Source: CAD feature listing. Evaluate the final solid. Frame: model axes, mm. Face numbers are marked on the shaded views. Coordinates: 2 decimals unless noted, no trailing zeros. Write each loop counter-clockwise with the first axis right and the second up, starting at its lowest first coordinate (ties: lowest second). Pieces come first, ordered by that corner, then holes. Notation, with made-up numbers: (-4, 56.25) -> (41, 56.25) arc R25 ccw to (41, 82.25) -> close; hole circle Ø6 at (79, 83). An arc over 180 degrees is marked (long way). One line per item, written item: value. Start each with the question number.
1. Line query: line 1 (Y direction, x = 0, z = 2.1); line 2 (X direction, y = -11, z = 0.5); line 3 (Z direction, x = 1.5, y = 17). Output: solid intervals per line, ascending.
2. Section query D-D, the plane x = 2.75. Output: boundary loops of the cut face in (y, z).
3. Section query B-B, the plane x = 0. Output: boundary loops of the cut face in (y, z).
4. Section query A-A, the plane y = 2.5. Output: boundary loops of the cut face in (x, z), and give its area (3 significant figures).
5. Mould query, pull axis X, two halves, no side actions, for the marked faces 1, 2 and 3. Classes: released by +X, released by -X, zero draft, split by the parting line, or undercut.
6. Section query C-C, the plane y = 9.5. Output: boundary loops of the cut face in (x, z), and give its area (3 significant figures).
from build123d import *

# Parameters (mm, degrees)
F0_W     = 25
F0_H     = 40
F1_DEPTH = 3
F2_W     = 11
F2_H     = 40
F3_DEPTH = 1.5
F4_R     = 2
F5_DEPTH = 3.001


with BuildPart() as f1:
    # F0 (on Top) → F1 (new body)
    with BuildSketch(Plane.XY):
        Rectangle(F0_W, F0_H)
    extrude(amount=F1_DEPTH)

    # F2 (on face) → F3 (cut)
    with BuildSketch(Plane(origin=(0, 0, 0), x_dir=(1, 0, 0), z_dir=(0, 0, -1))):
        Rectangle(F2_W, F2_H)
    extrude(amount=-F3_DEPTH, mode=Mode.SUBTRACT)

    # F4 (on face) → F5 (cut, through all)
    with BuildSketch(Plane.XY.offset(3)):
        with Locations((0, 2.5)):
            Circle(F4_R)
    extrude(amount=-F5_DEPTH, mode=Mode.SUBTRACT)


solid = f1.part
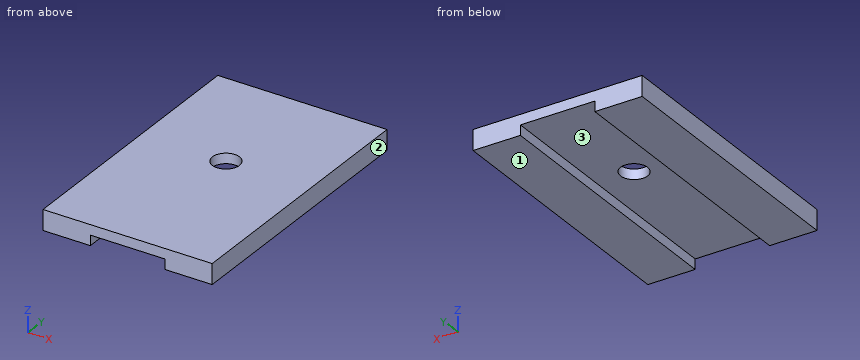
Computed values:
1. line 1: y = -20 to 0.5, 4.5 to 20
1. line 2: x = -12.5 to -5.5, 5.5 to 12.5
1. line 3: z = 1.5 to 3
2. outline: (-20, 1.5) -> (20, 1.5) -> (20, 3) -> (-20, 3) -> close
3. outline: (-20, 1.5) -> (0.5, 1.5) -> (0.5, 3) -> (-20, 3) -> close; (4.5, 1.5) -> (20, 1.5) -> (20, 3) -> (4.5, 3) -> close
4. outline: (-12.5, 0) -> (-5.5, 0) -> (-5.5, 1.5) -> (-2, 1.5) -> (-2, 3) -> (-12.5, 3) -> close; (2, 1.5) -> (5.5, 1.5) -> (5.5, 0) -> (12.5, 0) -> (12.5, 3) -> (2, 3) -> close
4. area: 52.5 mm²
5. face 1: zero draft
5. face 2: released by +X
5. face 3: undercut
6. outline: (-12.5, 0) -> (-5.5, 0) -> (-5.5, 1.5) -> (5.5, 1.5) -> (5.5, 0) -> (12.5, 0) -> (12.5, 3) -> (-12.5, 3) -> close
6. area: 58.5 mm²
